The model under review builds one solid part; all positions refer to its coordinate system, in mm. Face numbers are marked on the shaded views. A direction names the side the tool comes from. Coordinates: 2 decimals unless noted, no trailing zeros. Order: outer loops, then holes, each group sorted by start corner. A loop starts at its lowest first (then second) coordinate and runs counter-clockwise, first axis right, second up. Notation, with made-up numbers: (-22, 6) - (-12, 6) arc R23 ccw to (-12, 18) - close; hole circle Ø8 at (38.25, 48.25). An arc over 180 degrees is marked (long way). Answer in a Markdown table with one row per item.
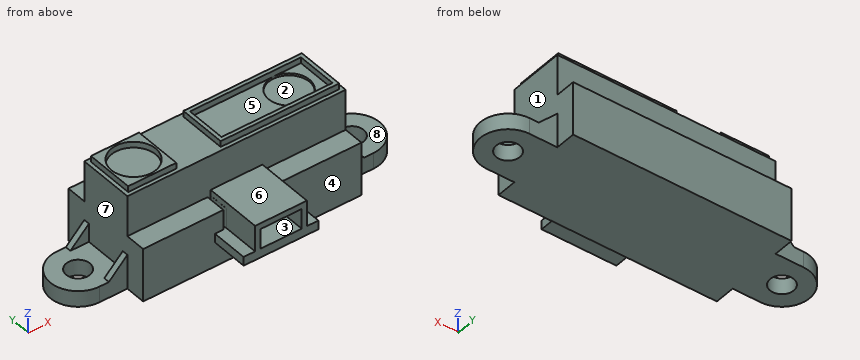
```python
from build123d import *

# Parameters (mm, degrees)
SKETCH_1_W          = 29.5
SKETCH_1_H          = 7.5
EXTRUDE_1_DEPTH     = 13.5
SKETCH_1_4_R        = 1.6
EXTRUDE_2_DEPTH     = 2.15
EXTRUDE_3_DEPTH     = 0.8
EXTRUDE_4_DEPTH     = 0.8
SKETCH_4_W          = 29.5
SKETCH_4_H          = 7.5
SKETCH_4_W_2        = 6.5
SKETCH_4_H_2        = 6.5
SKETCH_4_W_3        = 16
SKETCH_4_W_4        = 15
SKETCH_4_H_3        = 5.5
SKETCH_4_R          = 3
CUT_EXTRUDE_1_DEPTH = 0.8
SKETCH_7_W          = 29.5
SKETCH_7_H          = 13
EXTRUDE_5_DEPTH     = 7.2
SKETCH_10_W         = 10.1
SKETCH_10_H         = 1.2
SKETCH_10_W_2       = 7
SKETCH_10_H_2       = 2.7
SKETCH_10_H_3       = 0.8
EXTRUDE_7_DEPTH     = 7.75
SKETCH_11_W         = 5.595198372
SKETCH_11_H         = 2.7
SKETCH_11_W_2       = 0.4
CUT_EXTRUDE_2_DEPTH = 7.75
SKETCH_12_R         = 2.75
CUT_EXTRUDE_3_DEPTH = 0.3


with BuildPart() as part:
    # 草图1 → 凸台-拉伸1 (new body)
    with BuildSketch(Plane.XY):
        Rectangle(SKETCH_1_W, SKETCH_1_H)
    extrude(amount=EXTRUDE_1_DEPTH)

    # 草图1<4> → 凸台-拉伸2 (add)
    with BuildSketch(Plane.XY):
        with BuildLine():
            Line((-18.5, -3.75), (-14.75, -3.75))
            Line((-14.75, -3.75), (-14.75, 3.75))
            Line((-14.75, 3.75), (-18.5, 3.75))
            ThreePointArc((-18.5, 3.75), (-22.25, 0), (-18.5, -3.75))
        make_face()
        with Locations((-18.5, 0)):
            Circle(SKETCH_1_4_R, mode=Mode.SUBTRACT)
        with BuildLine():
            Line((14.75, -3.75), (18.5, -3.75))
            ThreePointArc((18.5, -3.75), (22.25, 0), (18.5, 3.75))
            Line((18.5, 3.75), (14.75, 3.75))
            Line((14.75, 3.75), (14.75, -3.75))
        make_face()
        with Locations((18.5, 0)):
            Circle(SKETCH_1_4_R, mode=Mode.SUBTRACT)
    extrude(amount=EXTRUDE_2_DEPTH)

    # 草图2 → 凸台-拉伸3 (add)
    with BuildSketch(Plane.XZ.offset(3.75)):
        Polygon((-14.75, 4.65), (-17.25, 2.15), (-14.75, 2.15), align=None)
        Polygon((14.75, 4.65), (17.25, 2.15), (14.75, 2.15), align=None)
    extrude(amount=-EXTRUDE_3_DEPTH)

    # 草图3 → 凸台-拉伸4 (add)
    with BuildSketch(Plane(origin=(0, 3.75, 0), x_dir=(1, 0, 0), z_dir=(0, 1, 0))):
        Polygon((17.25, -2.15), (14.75, -2.15), (14.75, -4.65), align=None)
        Polygon((-14.75, -4.65), (-14.75, -2.15), (-17.25, -2.15), align=None)
    extrude(amount=-EXTRUDE_4_DEPTH)

    # 草图4 → 切除-拉伸1 (cut)
    with BuildSketch(Plane.XY.offset(13.5)):
        Rectangle(SKETCH_4_W, SKETCH_4_H)
        with Locations((-11, 0)):
            Rectangle(SKETCH_4_W_2, SKETCH_4_H_2, mode=Mode.SUBTRACT)
        with Locations((6.25, 0)):
            Rectangle(SKETCH_4_W_3, SKETCH_4_H_2, mode=Mode.SUBTRACT)
        with Locations((6.25, 0)):
            Rectangle(SKETCH_4_W_4, SKETCH_4_H_3)
        with Locations((-11, 0)):
            Circle(SKETCH_4_R)
    extrude(amount=-CUT_EXTRUDE_1_DEPTH, mode=Mode.SUBTRACT)

    # 草图7 → 凸台-拉伸5 (add)
    with BuildSketch(Plane.XY):
        Rectangle(SKETCH_7_W, SKETCH_7_H)
    extrude(amount=EXTRUDE_5_DEPTH)

    # 草图10 → 凸台-拉伸7 (add)
    with BuildSketch(Plane.XZ.offset(3.75)):
        with Locations((0, 3.9)):
            Rectangle(SKETCH_10_W, SKETCH_10_H)
        with Locations((0, 5.85)):
            Rectangle(SKETCH_10_W_2, SKETCH_10_H_2)
        with Locations((0, 7.6)):
            Rectangle(SKETCH_10_W_2, SKETCH_10_H_3)
    extrude(amount=EXTRUDE_7_DEPTH)

    # 草图11 → 切除-拉伸2 (cut)
    with BuildSketch(Plane.XZ.offset(11.5)):
        with Locations((0, 5.85)):
            Rectangle(SKETCH_11_W, SKETCH_11_H)
        with Locations((3.7, 5.85)):
            Rectangle(SKETCH_11_W_2, SKETCH_11_H)
        with Locations((-3.707390598, 5.85)):
            Rectangle(SKETCH_11_W_2, SKETCH_11_H)
    extrude(amount=-CUT_EXTRUDE_2_DEPTH, mode=Mode.SUBTRACT)

    # 草图12 → 切除-拉伸3 (cut)
    with BuildSketch(Plane.XY.offset(12.7)):
        with Locations((10.011243367, 0)):
            Circle(SKETCH_12_R)
    extrude(amount=-CUT_EXTRUDE_3_DEPTH, mode=Mode.SUBTRACT)


solid = part.part
```
Item 1: We need section B-B, the plane x = -11. Write out the cut boundary in (y, z), then the cut area to 3 significant figures.
Check values:
| item | result |
|---|---|
| outline | (-6.5, 0) - (6.5, 0) - (6.5, 7.2) - (3.75, 7.2) - (3.75, 12.7) - (3.25, 12.7) - (3.25, 13.5) - (3, 13.5) - (3, 12.7) - (-3, 12.7) - (-3, 13.5) - (-3.25, 13.5) - (-3.25, 12.7) - (-3.75, 12.7) - (-3.75, 7.2) - (-6.5, 7.2) - close |
| area | 135 mm^2 |
Item 2: Tool access review of the marked faces 5, 6, 7 and 8: name each direction out of +Z, -Z, +X, -X, +Y, -Y from which nothing blocks a thin tool from reaching the whole face with its end or side.
Check values:
| item | result |
|---|---|
| face 5 | +Z |
| face 6 | +Z, +X, -X, -Y |
| face 7 | +Z, -X |
| face 8 | +Z, +X |
Item 3: Mouldability with a two-part tool opening along X and no side actions: class the marked faces 1, 2, 3 and 4 as +X half, -X half, draft (parallel to the pull), parting line (faces both ways), or undercut.
Check values:
| item | result |
|---|---|
| face 1 | +X half |
| face 2 | undercut |
| face 3 | undercut |
| face 4 | draft |
Item 4: We need section A-A, the plane z = 1.75. Write out the cut boundary in (x, y), then the cut area to 3 significant figures.
Check values:
| item | result |
|---|---|
| outline | (-18.5, -3.75) - (-14.75, -3.75) - (-14.75, -6.5) - (14.75, -6.5) - (14.75, -3.75) - (18.5, -3.75) arc R3.75 ccw to (18.5, 3.75) - (14.75, 3.75) - (14.75, 6.5) - (-14.75, 6.5) - (-14.75, 3.75) - (-18.5, 3.75) arc R3.75 ccw to start; hole circle Ø3.2 at (-18.5, 0); hole circle Ø3.2 at (18.5, 0) |
| area | 468 mm^2 |
Item 5: We need section D-D, the plane y = 5. Write out the cut boundary in (x, z), then the cut area to 3 significant figures.
Check values:
| item | result |
|---|---|
| outline | (-14.75, 0) - (14.75, 0) - (14.75, 7.2) - (-14.75, 7.2) - close |
| area | 212 mm^2 |
Item 6: To check wall thickness, follow line 1 (Y direction, x = -11, z = 13.15); line 2 (Y direction, x = -18.5, z = 1.6); line 3 (X direction, y = 0, z = 12.5). State the ranges of each line that lie inside material, in increasing order. Write a range as from..to.
Check values:
| item | result |
|---|---|
| line 1 | -3.25..-3, 3..3.25 |
| line 2 | -3.75..-1.6, 1.6..3.75 |
| line 3 | -14.75..7.26, 12.76..14.75 |
Item 7: We need section C-C, the plane y = 0. State how many separate pieces and enclosed holes the cut face has, then the cut area to 3 significant figures.
Check values:
| item | result |
|---|---|
| separate pieces | 3 |
| enclosed holes | 0 |
| area | 393 mm^2 |
Item 8: Clearance check with flat-ended pins moving along their axes: pin 1 Ø8 at (x, z) = (0.5, 7.5) entering from +Y; pin 2 Ø0.6 at (x, z) = (-12, 13.5) entering from -Y; pin 3 Ø3 at (x, y) = (-12, -1) entering from +Z; pin 4 Ø4 at (y, z) = (3, 8) entering from -X. State where each tip first meets the part, or that it passes through.
Check values:
| item | result |
|---|---|
| pin 1 | y = 6.5 |
| pin 2 | y = -3.25 |
| pin 3 | z = 12.7 |
| pin 4 | x = -14.75 |
